```python
from build123d import *

# Parameters (mm, degrees)
F0_W     = 10
F0_H     = 2
F1_DEPTH = 10


with BuildPart() as f1:
    # F0 (on Right) → F1 (new body)
    with BuildSketch(Plane.YZ):
        Polygon((10.5, -2.5), (10.5, 2.5), (-10.5, 2.5), (-10.5, -2.5), (-8.5, -2.5), (-8.5, 0.5), (-6, 0.5), (-6, 1.459846), (6, 1.459846), (6, 0.5), (8.5, 0.5), (8.5, -2.5), align=None)
        Polygon((6, -1.459846), (6, 0.5), (6, 1.459846), (-6, 1.459846), (-6, 0.5), (-6, -1.459846), align=None)
        Rectangle(F0_W, F0_H, mode=Mode.SUBTRACT)
    extrude(amount=F1_DEPTH)


solid = f1.part
```
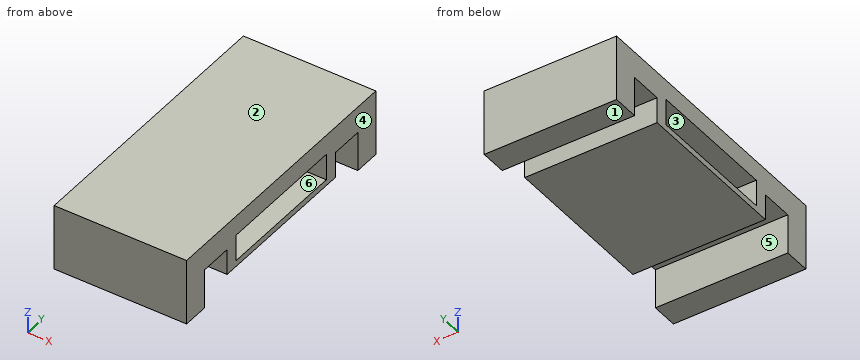
Input: part model. Units: mm. Frame: model coordinates. Face numbers are marked on the shaded views. A direction names the side the tool comes from. Give positions to 0.01 mm unless a question says otherwise; leave off trailing zeros. Loops run counter-clockwise (first coordinate to the right, second up) from the corner with the lowest first, then second, coordinate; pieces in that order, holes last. Notation, with made-up numbers: M -13.75,30.25 L 25.25,30.25 A22 ccw 25.25,67.25 Z; hole C 83.5,46 d6. An arc over 180 degrees is marked long. Answer as CSV lines item,"result". Start each with the question number.
1. Section C-C on z = -0.1. Return loops of the section in (x, y).
2. Pin query (flat end, axial travel): P1, Ø3, axis at x = 5, y = -1.5, coming from the -Z side. Return the tip coordinate at first contact, or that it passes through.
3. Reachability of the marked faces 4, 5 and 6 from +Z, -Z, +X, -X, +Y, -Y: full face, straight path, thin tool, end or side. Return the list, or none.
4. Line query: L1, parallel to Y at x = 6.5, z = -0.75; L2, parallel to Y at x = 8.5, z = -1.25; L3, parallel to Y at x = 9.5, z = -1.5. Output: solid intervals per line, ascending.
5. Section A-A on x = 7. Return loops of the section in (y, z), plus the area to 3 significant figures.
6. Pull-direction query (Z, two-part tool) for the marked faces 1, 2 and 3; classes: released by +Z, released by -Z, zero draft, split by the parting line, or undercut.
7. Section B-B on y = 0. Return loops of the section in (x, z).
8. Section D-D on y = 7.75. Return loops of the section in (x, z).
Computed values:
1,outline,"M 0,-10.5 L 10,-10.5 L 10,-8.5 L 0,-8.5 Z; M 0,-6 L 10,-6 L 10,-5 L 0,-5 Z; M 0,5 L 10,5 L 10,6 L 0,6 Z; M 0,8.5 L 10,8.5 L 10,10.5 L 0,10.5 Z"
2,P1,"stops at z = -1.46"
3,face 4,"+Z, -Z, +X, +Y, -Y"
3,face 5,"-Z, +X, -X"
3,face 6,"+X, -X"
4,L1,"y = -10.5 to -8.5, -6 to -5, 5 to 6, 8.5 to 10.5"
4,L2,"y = -10.5 to -8.5, -6 to 6, 8.5 to 10.5"
4,L3,"y = -10.5 to -8.5, 8.5 to 10.5"
5,outline,"M -10.5,-2.5 L -8.5,-2.5 L -8.5,0.5 L -6,0.5 L -6,-1.46 L 6,-1.46 L 6,0.5 L 8.5,0.5 L 8.5,-2.5 L 10.5,-2.5 L 10.5,2.5 L -10.5,2.5 Z; hole M -5,-1 L 5,-1 L 5,1 L -5,1 Z"
5,area,"57.5 mm²"
6,face 1,"released by -Z"
6,face 2,"released by +Z"
6,face 3,"undercut"
7,outline,"M 0,-1.46 L 10,-1.46 L 10,-1 L 0,-1 Z; M 0,1 L 10,1 L 10,2.5 L 0,2.5 Z"
8,outline,"M 0,0.5 L 10,0.5 L 10,2.5 L 0,2.5 Z"
